from build123d import *

# Parameters (mm, degrees)
F0_R     = 20
F1_DEPTH = 80
F3_W     = 40
F3_H     = 50
F4_DEPTH = 50
F5_R     = 12.5
F6_DEPTH = 20


with BuildPart() as f1:
    # F0 (on Front) → F1 (new body)
    with BuildSketch(Plane.XZ):
        Circle(F0_R)
    extrude(amount=F1_DEPTH)

    # F3 (on offset) → F4 (join)
    with BuildSketch(Plane.XZ.offset(15)):
        Rectangle(F3_W, F3_H)
    extrude(amount=F4_DEPTH)

    # F5 (on face) → F6 (cut)
    with BuildSketch(Plane.YZ.offset(20)):
        with Locations((-40, 0)):
            Circle(F5_R)
    extrude(amount=-F6_DEPTH, mode=Mode.SUBTRACT)


solid = f1.part
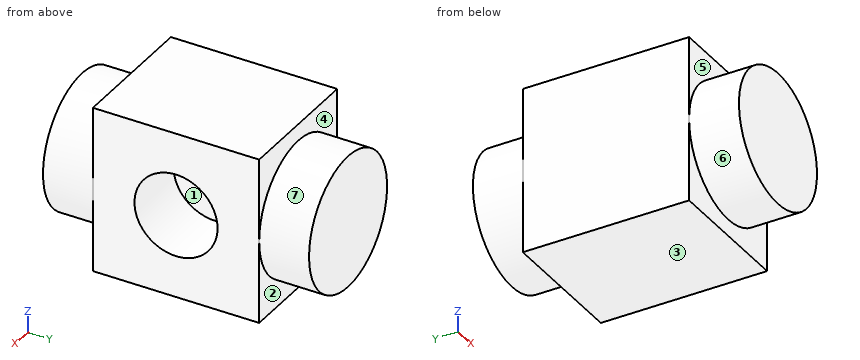
CAD build for the part. Positions are in the model's coordinates, mm. Face numbers are marked on the shaded views. A direction names the side the tool comes from. Round coordinates to 2 decimals unless told otherwise and drop trailing zeros. Write each loop counter-clockwise with the first axis right and the second up, starting at its lowest first coordinate (ties: lowest second). Pieces come first, ordered by that corner, then holes. Notation, with made-up numbers: M 28.5,16 L 70.5,16 A25 ccw 70.5,45 Z; hole C 38,2.5 d3. An arc over 180 degrees is marked long. Put each result on its own line as item: value. Start each with the question number.
1) Pull direction Y, two halves, no side cores. Call the marked faces 1, 2 and 3: pulls with the +Y half, pulls with the -Y half, needs draft (parallel to the pull), parting line crosses it, or undercut.
2) Saw through at A-A, the plane y = -40. Write the cut outline in (x, z), and give its area (3 significant figures).
3) Saw through at C-C, the plane x = -13.5. Write the cut outline in (y, z).
4) Drill centre lines: probe 1 along Z at (x, y) = (13, -40); probe 2 along Z at (x, y) = (-0.5, -74); probe 3 along Y at (x, z) = (-15.5, -16.5). Where is each one in solid material? Low to high. Write a range as [from, to].
5) Saw through at D-D, the plane x = 11.5. Write the cut outline in (y, z), and give its area (3 significant figures).
6) Saw through at B-B, the plane z = 16. Write the cut outline in (x, y), and give its area (3 significant figures).
7) 3-axis set-ups, long thin cutter, end or side, ignore diameter. For the marked faces 4, 5, 6 and 7: which of +Z, -Z, +X, -X, +Y, -Y reach the whole face in a straight line?
8) Pin check, flat tip, straight feed: pin 1 Ø7.5 at (y, z) = (-44, 1.5) entering from +X. Stop position of the tip, or through.
Resolved:
1. face 1: undercut
1. face 2: pulls with the +Y half
1. face 3: needs draft
2. outline: M -20,-25 L 20,-25 L 20,-12.5 L 0,-12.5 L 0,12.5 L 20,12.5 L 20,25 L -20,25 Z
2. area: 1,500 mm²
3. outline: M -80,-14.76 L -65,-14.76 L -65,-25 L -15,-25 L -15,-14.76 L 0,-14.76 L 0,14.76 L -15,14.76 L -15,25 L -65,25 L -65,14.76 L -80,14.76 Z
4. probe 1: [-25, -12.5], [12.5, 25]
4. probe 2: [-19.99, 19.99]
4. probe 3: [-65, -15]
5. outline: M -80,-16.36 L -65,-16.36 L -65,-25 L -15,-25 L -15,-16.36 L 0,-16.36 L 0,16.36 L -15,16.36 L -15,25 L -65,25 L -65,16.36 L -80,16.36 Z; hole C -40,0 d25
5. area: 2,990 mm²
6. outline: M -20,-65 L -12,-65 L -12,-80 L 12,-80 L 12,-65 L 20,-65 L 20,-15 L 12,-15 L 12,0 L -12,0 L -12,-15 L -20,-15 Z
6. area: 2,720 mm²
7. face 4: +Z, +Y
7. face 5: +Z, -Y
7. face 6: -Y
7. face 7: +Y
8. pin 1: x = 0
